For this review, take the finished solid that the model builds, in its own axes (mm). A direction names the side the tool comes from. Round coordinates to 2 decimals unless told otherwise and drop trailing zeros. Order: outer loops, then holes, each group sorted by start corner. A loop starts at its lowest first (then second) coordinate and runs counter-clockwise, first axis right, second up. Notation, with made-up numbers: (43.25, 51) -> (64.25, 51) arc R30 cw to (64.25, 87) -> close; hole circle Ø5 at (67.5, -7). An arc over 180 degrees is marked (long way). Answer in a Markdown table with one row per item.
```python
from build123d import *

# Parameters (mm, degrees)
F1_DEPTH = 76.2
F2_W     = 76.2
F2_H     = 25.4
F3_DEPTH = 76.2


with BuildPart() as f1:
    # F0 (on Front) → F1 (new body)
    with BuildSketch(Plane.XZ):
        Polygon((-76.2, 25.4), (-76.2, 0), (76.2, 0), (76.2, 25.4), (0, 25.4), align=None)
    extrude(amount=F1_DEPTH)

    # F2 (on Front) → F3 (join)
    with BuildSketch(Plane.XZ):
        with Locations((-38.1, 37.732552)):
            Rectangle(F2_W, F2_H)
    extrude(amount=F3_DEPTH)


solid = f1.part
```
Q1. Take a section at A-A, the plane y = -38. Write out the cut boundary in (x, z), then the cut area to 3 significant figures.
Answer key:
| item | result |
|---|---|
| outline | (-76.2, 0) -> (76.2, 0) -> (76.2, 25.4) -> (0, 25.4) -> (0, 50.43) -> (-76.2, 50.43) -> close |
| area | 5,780 mm^2 |
Q2. Tool access review of faces 1 (the face through (-1, -38, 0)), 2 (the face through (39, -38, 25.4)): name each direction out of +Z, -Z, +X, -X, +Y, -Y from which nothing blocks a thin tool from reaching the whole face with its end or side.
Answer key:
| item | result |
|---|---|
| face 1 | -Z, +X, -X, +Y, -Y |
| face 2 | +Z, +X, +Y, -Y |
Q3. Clearance check with a flat-ended pin moving along its axis: pin 1 Ø20 at (y, z) = (-40, 42.5) entering from +X. State where the tip first meets the part, or that it passes through.
Answer key:
| item | result |
|---|---|
| pin 1 | stops at x = 0 |
Q4. To check wall thickness, follow probe 1 along Z at (x, y) = (31, -2.5); probe 2 along X at (y, z) = (-36.5, 33). State the ranges of each line that lie inside material, in increasing order.
Answer key:
| item | result |
|---|---|
| probe 1 | z = 0 to 25.4 |
| probe 2 | x = -76.2 to 0 |
Q5. Take a section at B-B, the plane z = 34.5. Write out the cut boundary in (x, y).
Answer key:
| item | result |
|---|---|
| outline | (-76.2, -76.2) -> (0, -76.2) -> (0, 0) -> (-76.2, 0) -> close |
